CAD build for the part. Positions are in the model's coordinates, mm. A direction names the side the tool comes from. Give positions to 0.01 mm unless a question says otherwise; leave off trailing zeros. Order: outer loops, then holes, each group sorted by start corner. A loop starts at its lowest first (then second) coordinate and runs counter-clockwise, first axis right, second up.
Item 1: Flat gauge pins, fed straight in: P1, Ø5, axis at x = 6, z = 12, coming from the -Y side; P2, Ø1.5, axis at x = 4.5, z = 40.5, coming from the +Y side; P3, Ø22.5, axis at y = 1.83, z = -14.52, coming from the +X side. Where does each tip first touch, or does it go through?
Item 2: Band-saw the part on B-B on z = -45. Give the cut face in (x, y), plus the area to 3 significant figures.
Item 3: Band-saw the part on A-A on y = -8.5. Give the cut face in (x, z), plus the area to 3 significant figures.
Item 4: Wall check: L1, parallel to Y at x = 7.75, z = -9; L2, parallel to Z at x = 3.25, y = -7; L3, parallel to Z at x = 6.25, y = -4.5. Give the ranges that are in metal, low to high.
Item 5: Which spindle directions (+Z, -Z, +X, -X, +Y, -Y) get a long thin tool onto all of the face, cutting with end or side? Do faces 1 (the flat face through (6.26, -50.21, 46.65)), 2 (the cylindrical face through (6.44, -0.9, -26.82)), 3 (the flat face through (6.3, -20, -68.6)). Say none if no direction does.
Item 6: Two-plate mould, pull along Z, no slides. Class faces 4 (the flat face through (0, -15, -23)), 5 (the flat face through (6.3, -46.4, -31.4)), 6 (the flat face through (6.261, 45.04, -64.596)): released by +Z, released by -Z, zero draft, split by the parting line, or undercut.
Item 7: Band-saw the part on C-C on y = 47. Give the cut face in (x, z), plus the area to 3 significant figures.
```python
from build123d import *

# Parameters (mm, degrees)
F1_DEPTH = 12.7
F2_R     = 12.5952384753
F3_DEPTH = 12.7


with BuildPart() as f1:
    # F0 (on Right) → F1 (new body)
    with BuildSketch(Plane.YZ):
        with BuildLine():
            add(Edge.make_bspline(
                [(-57.3755726218, 60.9794743359), (-50.213151662, 55.4152866858), (-37.2366697029, 55.7418096569), (-31.8573741668, 63.5785382982), (-31.6838938743, 72.6575106382)],
                knots=[0, 0, 0, 0, 0.5161301104, 1, 1, 1, 1], degree=3))
            Line((-57.3755726218, 60.9794743359), (-42.8429059684, 31.9141410291))
            add(Edge.make_bspline(
                [(-36.2667675946, 0), (-34.2304695223, 4.5985213525), (-31.3995907567, 13.0121996142), (-40.343719866, 22.6597812459), (-42.8429059684, 31.9141410291)],
                knots=[0, 0, 0, 0, 0.4287022635, 1, 1, 1, 1], degree=3))
            Line((-36.2667675946, 0), (-56.8240570945, -63.699272458))
            add(Edge.make_bspline(
                [(-33.9242853224, -84.9647447467), (-31.6925561956, -70.080335482), (-35.9990572627, -60.9174321222), (-42.6189227408, -61.5948104869), (-56.8240570945, -63.699272458)],
                knots=[0, 0, 0, 0, 0.51017927, 1, 1, 1, 1], degree=3))
            Line((-33.9242853224, -84.9647447467), (-5.7011889294, -51.7937131226))
            add(Edge.make_bspline(
                [(10.6406565756, -54.0301650763), (6.3823924594, -52.4609805374), (-1.6627763206, -48.6585438271), (-0.9598822639, -49.5478302166), (-5.7011889294, -51.7937131226)],
                knots=[0, 0, 0, 0, 0.5787981071, 1, 1, 1, 1], degree=3))
            Line((10.6406565756, -54.0301650763), (80.4164707661, -75.4625424743))
            add(Edge.make_bspline(
                [(92.4523919821, -49.5390184224), (84.5183726601, -50.3969736232), (76.2899942249, -55.1051300096), (76.3544072931, -67.5799232364), (80.4164707661, -75.4625424743)],
                knots=[0, 0, 0, 0, 0.4758961852, 1, 1, 1, 1], degree=3))
            Line((92.4523919821, -49.5390184224), (44.148941397, -19.6030026067))
            add(Edge.make_bspline(
                [(19.77852609, 8.4459672519), (21.4932358048, 1.7455546836), (29.8932683418, -5.0282844876), (37.5500863975, -17.1425788423), (44.148941397, -19.6030026067)],
                knots=[0, 0, 0, 0, 0.4824482884, 1, 1, 1, 1], degree=3))
            Line((19.77852609, 8.4459672519), (-31.6838938743, 72.6575106382))
        make_face()
    extrude(amount=F1_DEPTH)

    # F2 (on face) → F3 (cut)
    with BuildSketch(Plane.YZ.offset(12.7)):
        with Locations((1.8296902999, -14.5234484226)):
            Circle(F2_R)
    extrude(amount=-F3_DEPTH, mode=Mode.SUBTRACT)


solid = f1.part
```
The answers:
1. P1: stops at y = -34.83
1. P2: stops at y = -5.31
1. P3: passes through
2. outline: (0, -50.79) - (12.7, -50.79) - (12.7, 85.13) - (0, 85.13) - close
2. area: 1,730 mm2
3. outline: (0, -55.08) - (12.7, -55.08) - (12.7, -21.73) - (0, -21.73) - close; (0, -7.32) - (12.7, -7.32) - (12.7, 43.73) - (0, 43.73) - close
3. area: 1,070 mm2
4. L1: y = -39.17 to -9.49, 13.15 to 31.87
4. L2: z = -53.32 to -23.51, -5.54 to 41.86
4. L3: z = -51.21 to -25.41, -3.63 to 38.74
5. face 1: +X, -X, -Y
5. face 2: +X, -X
5. face 3: -Z, +X, -X
6. face 4: zero draft
6. face 5: undercut
6. face 6: released by -Z
7. outline: (0, -65.2) - (12.7, -65.2) - (12.7, -21.37) - (0, -21.37) - close
7. area: 557 mm2
